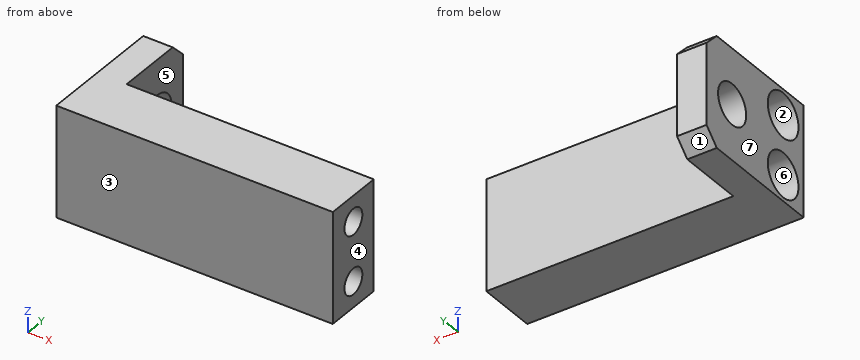
from build123d import *

# Parameters (mm, degrees)
BOSS_EXTRUDE1_DEPTH = 15
SKETCH2_R           = 2.75
SKETCH2_R_2         = 3
SKETCH2_R_3         = 1.75
CUT_EXTRUDE1_DEPTH  = 15
SKETCH3_R           = 1.75
CUT_EXTRUDE2_DEPTH  = 38.5
CHAMFER1_SIZE       = 2


with BuildPart() as part:
    # Sketch1 → Boss-Extrude1 (new body)
    with BuildSketch(Plane.XY):
        Polygon((-12.163709917, 2.060150376), (-8.163709917, 2.060150376), (-8.163709917, -8.939849624), (25.336290083, -8.939849624), (25.336290083, -16.939849624), (-12.163709917, -16.939849624), align=None)
    extrude(amount=BOSS_EXTRUDE1_DEPTH)

    # Sketch2 → Cut-Extrude1 (cut)
    with BuildSketch(Plane.ZY.offset(12.163709917)):
        with Locations((7.5, -2.939849624)):
            Circle(SKETCH2_R)
        with Locations((11.5, -12.914706032)):
            Circle(SKETCH2_R_2)
        with Locations((11.5, -12.914706032)):
            Circle(SKETCH2_R_3, mode=Mode.SUBTRACT)
        with Locations((3.5, -12.914706032)):
            Circle(SKETCH2_R_2)
        with Locations((3.5, -12.914706032)):
            Circle(SKETCH2_R_3, mode=Mode.SUBTRACT)
    extrude(amount=-CUT_EXTRUDE1_DEPTH, mode=Mode.SUBTRACT)

    # Sketch3 → Cut-Extrude2 (cut, through all)
    with BuildSketch(Plane.ZY.offset(12.163709917)):
        with Locations((3.5, -12.914706032)):
            Circle(SKETCH3_R)
        with Locations((11.5, -12.914706032)):
            Circle(SKETCH3_R)
    extrude(amount=-CUT_EXTRUDE2_DEPTH, mode=Mode.SUBTRACT)

    # Chamfer1
    chamfer1_edges = [part.edges().sort_by_distance(p)[0] for p in [
        (-10.163709917, 2.060150376, 15),
        (-10.163709917, 2.060150376, 0),
    ]]
    chamfer(chamfer1_edges, length=CHAMFER1_SIZE)


solid = part.part
Build history of the part. All positions in model axes, mm. Face numbers are marked on the shaded views. A direction names the side the tool comes from. Round coordinates to 2 decimals unless told otherwise and drop trailing zeros. Loops run counter-clockwise (first coordinate to the right, second up) from the corner with the lowest first, then second, coordinate; pieces in that order, holes last. Notation, with made-up numbers: (-28.75, 44) -> (19.25, 44) arc R9 ccw to (19.25, 50) -> close; hole circle Ø11 at (-16, -31). An arc over 180 degrees is marked (long way). Use CSV: the item, a comma, the result in double quotes. Start each with the question number.
Q1. Which spindle directions (+Z, -Z, +X, -X, +Y, -Y) get a long thin tool onto all of the face, cutting with end or side? Do the marked faces 5, 6 and 7. Say none if no direction does.
Q2. Saw through at B-B on y = -1.5. Give the cut face in (x, z), and give its area (3 significant figures).
Q3. Saw through at D-D on z = 7.5. Give the cut face in (x, y).
Q4. Flat gauge pins, fed straight in: pin 1 Ø4 at (x, z) = (-2.5, 9) entering from +Y; pin 2 Ø5.5 at (y, z) = (-12.91, 3.5) entering from -X. Where does each tip first touch, or does it go through?
Q5. Saw through at A-A on z = 3.5. Give the cut face in (x, y).
Q6. Drill centre lines: L1, parallel to Y at x = 13, z = 3.5; L2, parallel to Y at x = -8, z = 3.5; L3, parallel to Z at x = 9.5, y = -14.5. Where is each one in solid material? Low to high.
Q7. Mould opens along Y. For the marked faces 1, 2, 3 and 4 say: +Y half, -Y half, draft (parallel to the pull), parting line (faces both ways), or undercut.
Q8. Saw through at C-C on y = -12.5. Give the cut face in (x, z).
Solutions:
1,face 5,"+Z, -Z, +X, +Y"
1,face 6,"-X"
1,face 7,"+Z, -Z, -X, +Y, -Y"
2,outline,"(-12.16, 0) -> (-8.16, 0) -> (-8.16, 5.16) -> (-12.16, 5.16) -> close; (-12.16, 9.84) -> (-8.16, 9.84) -> (-8.16, 15) -> (-12.16, 15) -> close"
2,area,"41.3 mm^2"
3,outline,"(-12.16, -16.94) -> (25.34, -16.94) -> (25.34, -8.94) -> (-8.16, -8.94) -> (-8.16, -5.69) -> (-12.16, -5.69) -> close; (-12.16, -0.19) -> (-8.16, -0.19) -> (-8.16, 2.06) -> (-12.16, 2.06) -> close"
4,pin 1,"stops at y = -8.94"
4,pin 2,"stops at x = 2.84"
5,outline,"(-12.16, -16.94) -> (25.34, -16.94) -> (25.34, -14.66) -> (2.84, -14.66) -> (2.84, -15.91) -> (-12.16, -15.91) -> close; (-12.16, -9.91) -> (2.84, -9.91) -> (2.84, -11.16) -> (25.34, -11.16) -> (25.34, -8.94) -> (-8.16, -8.94) -> (-8.16, 2.06) -> (-12.16, 2.06) -> close"
6,L1,"y = -16.94 to -14.66, -11.16 to -8.94"
6,L2,"y = -16.94 to -15.91, -9.91 to -8.94"
6,L3,"z = 0 to 2.76, 4.24 to 10.76, 12.24 to 15"
7,face 1,"+Y half"
7,face 2,"undercut"
7,face 3,"-Y half"
7,face 4,"draft"
8,outline,"(-12.16, 0) -> (25.34, 0) -> (25.34, 1.8) -> (2.84, 1.8) -> (2.84, 0.53) -> (-12.16, 0.53) -> close; (-12.16, 6.47) -> (2.84, 6.47) -> (2.84, 5.2) -> (25.34, 5.2) -> (25.34, 9.8) -> (2.84, 9.8) -> (2.84, 8.53) -> (-12.16, 8.53) -> close; (-12.16, 14.47) -> (2.84, 14.47) -> (2.84, 13.2) -> (25.34, 13.2) -> (25.34, 15) -> (-12.16, 15) -> close"
